Can you work these out from the model? Positions are in its coordinate system, mm. A direction names the side the tool comes from. Give positions to 0.01 mm unless a question says otherwise; leave off trailing zeros. Write each loop counter-clockwise with the first axis right and the second up, starting at its lowest first coordinate (ties: lowest second). Pieces come first, ordered by that corner, then holes. Notation, with made-up numbers: (22, 38.5) - (64, 38.5) arc R18 cw to (64, 60.5) - close; hole circle Ø2 at (-9, -10.75). An arc over 180 degrees is marked (long way). Use a Markdown table: item, result. Add a question column.
```python
from build123d import *

# Parameters (mm, degrees)
EXTRUDE_1_DEPTH     = 2.5
SKETCH_2_R          = 4.064
SKETCH_2_R_2        = 2.54
EXTRUDE_2_DEPTH     = 3.75
SKETCH_3_R          = 18.887467654
SKETCH_3_R_2        = 12
CUT_EXTRUDE_3_DEPTH = 23.225268927


with BuildPart() as part:
    # Эскиз1 → Вытянуть1 (new body)
    with BuildSketch(Plane(origin=(0, 0, 0), x_dir=(1, 0, 0), z_dir=(0, 1, 0))):
        with BuildLine():
            Line((-1.842046714, -14.157953286), (-2.855725348, -7.29719043))
            ThreePointArc((-2.855725348, -7.29719043), (-3.589616048, -6.217397374), (-4.891689614, -6.121725913))
            Line((-4.891689614, -6.121725913), (-11.340123854, -8.674235892))
            ThreePointArc((-11.340123854, -8.674235892), (-13.856406461, -8), (-13.182170568, -5.483717394))
            Line((-13.182170568, -5.483717394), (-7.747414963, -1.175464517))
            ThreePointArc((-7.747414963, -1.175464517), (-7.179232096, 0), (-7.747414963, 1.175464517))
            Line((-7.747414963, 1.175464517), (-13.182170568, 5.483717394))
            ThreePointArc((-13.182170568, 5.483717394), (-13.856406461, 8), (-11.340123854, 8.674235892))
            Line((-11.340123854, 8.674235892), (-4.891689614, 6.121725913))
            ThreePointArc((-4.891689614, 6.121725913), (-3.589616048, 6.217397374), (-2.855725348, 7.29719043))
            Line((-2.855725348, 7.29719043), (-1.842046714, 14.157953286))
            ThreePointArc((-1.842046714, 14.157953286), (0, 16), (1.842046714, 14.157953286))
            Line((1.842046714, 14.157953286), (2.855725348, 7.29719043))
            ThreePointArc((2.855725348, 7.29719043), (3.589616048, 6.217397374), (4.891689614, 6.121725913))
            Line((4.891689614, 6.121725913), (11.340123854, 8.674235892))
            ThreePointArc((11.340123854, 8.674235892), (13.856406461, 8), (13.182170568, 5.483717394))
            Line((13.182170568, 5.483717394), (7.747414963, 1.175464517))
            ThreePointArc((7.747414963, 1.175464517), (7.179232096, 0), (7.747414963, -1.175464517))
            Line((7.747414963, -1.175464517), (13.182170568, -5.483717394))
            ThreePointArc((13.182170568, -5.483717394), (13.856406461, -8), (11.340123854, -8.674235892))
            Line((11.340123854, -8.674235892), (4.891689614, -6.121725913))
            ThreePointArc((4.891689614, -6.121725913), (3.589616048, -6.217397374), (2.855725348, -7.29719043))
            Line((2.855725348, -7.29719043), (1.842046714, -14.157953286))
            ThreePointArc((1.842046714, -14.157953286), (0, -16), (-1.842046714, -14.157953286))
        make_face()
    extrude(amount=EXTRUDE_1_DEPTH)

    # Эскиз2 → Вытянуть2 (add)
    with BuildSketch(Plane.XZ):
        with Locations(Location((0, 0, 0), (0, 0, 90))):
            Circle(SKETCH_2_R)
        with Locations(Location((0, 0, 0), (0, 0, 270))):
            Circle(SKETCH_2_R_2, mode=Mode.SUBTRACT)
    extrude(amount=EXTRUDE_2_DEPTH)

    # Эскиз3 → Вытянуть3 (cut, through all)
    with BuildSketch(Plane(origin=(0, 2.5, 0), x_dir=(-1, 0, 0), z_dir=(0, 1, 0))):
        Circle(SKETCH_3_R)
        Circle(SKETCH_3_R_2, mode=Mode.SUBTRACT)
    extrude(amount=-CUT_EXTRUDE_3_DEPTH, mode=Mode.SUBTRACT)


solid = part.part
```
Q1. I'm going to push flat-ended pins straight in: P1, Ø1.5, axis at y = 0, z = -1, coming from the -X side; P2, Ø5, axis at x = 7.5, z = 6, coming from the -Y side; P3, Ø2, axis at x = 2.5, y = 0, coming from the +Z side. Where does each tip first touch, or does it pass through?
Q2. If we mould it in two halves opening along Z, with no side actions, what happens to faces 6 (the cylindrical face through (3.967, -1.849, -0.881)), 7 (the cylindrical face through (2.52, -1.85, 0.33)), 8 (the flat face through (-5, 0, 0))? For each: released by +Z, released by -Z, zero draft, split by the parting line, or undercut.
Q3. Suppose I cut it at B-B (y = -1). Please give me the cut outline in (x, z).
Q4. Suppose I cut it at A-A (z = 0). Please give me the cut outline in (x, y).
Q5. Suppose I cut it at C-C (x = 0). Please give me the cut outline in (y, z).
Q6. If I drill on probe 1 along X at (y, z) = (-1.85, 0); probe 2 along Y at (x, z) = (-7.5, -1); probe 3 along Z at (x, y) = (-0.25, 1.5), over which ranges is the centre line in solid material (lowest first)? Write a range as [from, to].
Q7. On a 3-axis mill with a long thin cutter (end or side, diameter ignored), from which of +Z, -Z, +X, -X, +Y, -Y can I reach the whole of each face in a straight line? I mean faces 1 (the flat face through (9.56, 1.23, -2.61)), 2 (the flat face through (0, 2.5, 0)), 3 (the flat face through (-7.04, 1.23, -6.97)), 4 (the flat face through (7.04, 1.23, 6.97)), 5 (the flat face through (-9.56, 1.23, 2.61)). Say none if no direction works.
Q8. Suppose I cut it at D-D (y = 1.5). Please give me the cut outline in (x, z).
Derived:
| question | item | result |
|---|---|---|
| 1 | P1 | x = -8.47 |
| 1 | P2 | y = 0 |
| 1 | P3 | z = 11.91 |
| 2 | face 6 | split by the parting line |
| 2 | face 7 | undercut |
| 2 | face 8 | zero draft |
| 3 | outline | circle Ø8.13 at (0, 0); hole circle Ø5.08 at (0, 0) |
| 4 | outline | (-7.18, 0) - (-4.06, 0) - (-4.06, -3.75) - (-2.54, -3.75) - (-2.54, 0) - (2.54, 0) - (2.54, -3.75) - (4.06, -3.75) - (4.06, 0) - (7.18, 0) - (7.18, 2.5) - (-7.18, 2.5) - close |
| 5 | outline | (-3.75, -4.06) - (0, -4.06) - (0, -12) - (2.5, -12) - (2.5, 12) - (0, 12) - (0, 4.06) - (-3.75, 4.06) - (-3.75, 2.54) - (0, 2.54) - (0, -2.54) - (-3.75, -2.54) - close |
| 6 | probe 1 | [-4.06, -2.54], [2.54, 4.06] |
| 6 | probe 2 | [0, 2.5] |
| 6 | probe 3 | [-12, 12] |
| 7 | face 1 | +X, +Y, -Y |
| 7 | face 2 | +Z, -Z, +X, -X, +Y |
| 7 | face 3 | -Z, +Y, -Y |
| 7 | face 4 | +Z, +Y, -Y |
| 7 | face 5 | -X, +Y, -Y |
| 8 | outline | (-11.31, -4) arc R12 ccw to (-9.12, -7.8) - (-4.89, -6.12) arc R1.5 cw to (-2.86, -7.3) - (-2.19, -11.8) arc R12 ccw to (2.19, -11.8) - (2.86, -7.3) arc R1.5 cw to (4.89, -6.12) - (9.12, -7.8) arc R12 ccw to (11.31, -4) - (7.75, -1.18) arc R1.5 cw to (7.75, 1.18) - (11.31, 4) arc R12 ccw to (9.12, 7.8) - (4.89, 6.12) arc R1.5 cw to (2.86, 7.3) - (2.19, 11.8) arc R12 ccw to (-2.19, 11.8) - (-2.86, 7.3) arc R1.5 cw to (-4.89, 6.12) - (-9.12, 7.8) arc R12 ccw to (-11.31, 4) - (-7.75, 1.18) arc R1.5 cw to (-7.75, -1.18) - close |
